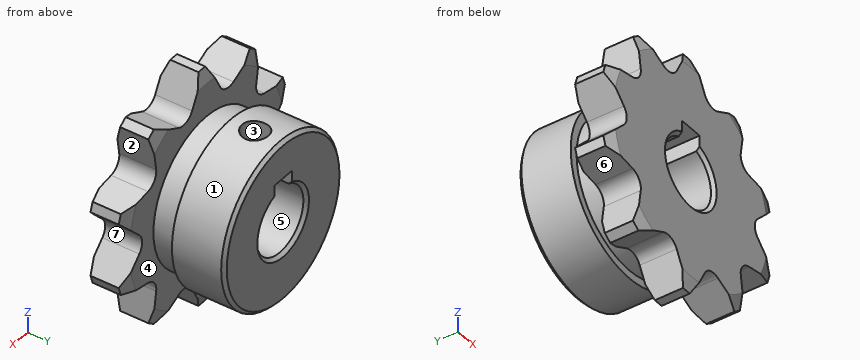
from build123d import *

# Parameters (mm, degrees)
SALIENTE_EXTRUIR1_DEPTH = 7.2136
CROQUIS2_R              = 15.875
SALIENTE_EXTRUIR2_DEPTH = 15.0114
CROQUIS5_R              = 6.35
CORTAR_EXTRUIR2_DEPTH   = 23.2250001
CHAFL_N2_SIZE           = 0.635
REDONDEO1_R             = 0.635
CROQUIS8_W              = 3.175
CROQUIS8_H              = 4.7625
CROQUIS9_W              = 2.5527
CROQUIS9_H              = 15.875
CHAFL_N3_SIZE           = 0.635
CROQUIS11_W             = 4.7625
CROQUIS11_H             = 4.7625
CORTAR_EXTRUIR3_DEPTH   = 23.225


with BuildPart() as part:
    # Croquis1 → Saliente-Extruir1 (new body)
    with BuildSketch(Plane(origin=(0, 0, 0), x_dir=(1, 0, 0), z_dir=(0, 1, 0))):
        with BuildLine():
            Line((12.977610276, 19.417818353), (7.368467037, 16.623783971))
            ThreePointArc((7.368467037, 16.623783971), (5.352847667, 16.474371141), (3.81, 17.78))
            Line((3.81, 17.78), (0.9144, 23.337392972))
            ThreePointArc((0.9144, 23.337392972), (0, 23.3553), (-0.9144, 23.337392972))
            Line((-0.9144, 23.337392972), (-3.81, 17.78))
            ThreePointArc((-3.81, 17.78), (-5.352847667, 16.474371141), (-7.368467037, 16.623783971))
            Line((-7.368467037, 16.623783971), (-12.977610276, 19.417818353))
            ThreePointArc((-12.977610276, 19.417818353), (-13.727900903, 18.894834609), (-14.457140556, 18.342876684))
            Line((-14.457140556, 18.342876684), (-13.533176534, 12.144860349))
            ThreePointArc((-13.533176534, 12.144860349), (-14.013937128, 10.181721309), (-15.732430111, 9.117847487))
            Line((-15.732430111, 9.117847487), (-21.91261452, 8.081297111))
            ThreePointArc((-21.91261452, 8.081297111), (-22.212210255, 7.217184609), (-22.477744799, 6.342004954))
            Line((-22.477744799, 6.342004954), (-18.087139608, 1.870796833))
            ThreePointArc((-18.087139608, 1.870796833), (-17.322178923, 0), (-18.087139608, -1.870796833))
            Line((-18.087139608, -1.870796833), (-22.477744799, -6.342004954))
            ThreePointArc((-22.477744799, -6.342004954), (-22.212210255, -7.217184609), (-21.91261452, -8.081297111))
            Line((-21.91261452, -8.081297111), (-15.732430111, -9.117847487))
            ThreePointArc((-15.732430111, -9.117847487), (-14.013937128, -10.181721309), (-13.533176534, -12.144860349))
            Line((-13.533176534, -12.144860349), (-14.457140556, -18.342876684))
            ThreePointArc((-14.457140556, -18.342876684), (-13.727900903, -18.894834609), (-12.977610276, -19.417818353))
            Line((-12.977610276, -19.417818353), (-7.368467037, -16.623783971))
            ThreePointArc((-7.368467037, -16.623783971), (-5.352847667, -16.474371141), (-3.81, -17.78))
            Line((-3.81, -17.78), (-0.9144, -23.337392972))
            ThreePointArc((-0.9144, -23.337392972), (0, -23.3553), (0.9144, -23.337392972))
            Line((0.9144, -23.337392972), (3.81, -17.78))
            ThreePointArc((3.81, -17.78), (5.352847667, -16.474371141), (7.368467037, -16.623783971))
            Line((7.368467037, -16.623783971), (12.977610276, -19.417818353))
            ThreePointArc((12.977610276, -19.417818353), (13.727900903, -18.894834609), (14.457140556, -18.342876684))
            Line((14.457140556, -18.342876684), (13.533176534, -12.144860349))
            ThreePointArc((13.533176534, -12.144860349), (14.013937128, -10.181721309), (15.732430111, -9.117847487))
            Line((15.732430111, -9.117847487), (21.91261452, -8.081297111))
            ThreePointArc((21.91261452, -8.081297111), (22.212210255, -7.217184609), (22.477744799, -6.342004954))
            Line((22.477744799, -6.342004954), (18.087139608, -1.870796833))
            ThreePointArc((18.087139608, -1.870796833), (17.322178923, 0), (18.087139608, 1.870796833))
            Line((18.087139608, 1.870796833), (22.477744799, 6.342004954))
            ThreePointArc((22.477744799, 6.342004954), (22.212210255, 7.217184609), (21.91261452, 8.081297111))
            Line((21.91261452, 8.081297111), (15.732430111, 9.117847487))
            ThreePointArc((15.732430111, 9.117847487), (14.013937128, 10.181721309), (13.533176534, 12.144860349))
            Line((13.533176534, 12.144860349), (14.457140556, 18.342876684))
            ThreePointArc((14.457140556, 18.342876684), (13.727900903, 18.894834609), (12.977610276, 19.417818353))
        make_face()
    extrude(amount=SALIENTE_EXTRUIR1_DEPTH)

    # Croquis2 → Saliente-Extruir2 (add)
    with BuildSketch(Plane(origin=(0, 7.2136, 0), x_dir=(1, 0, 0), z_dir=(0, 1, 0))):
        Circle(CROQUIS2_R)
    extrude(amount=SALIENTE_EXTRUIR2_DEPTH)

    # Croquis3 → Cortar-Revolución3 (revolve, cut)
    with BuildSketch(Plane(origin=(0, 0, 0), x_dir=(0, 0, -1), z_dir=(1, 0, 0))):
        Polygon((23.972392972, 7.2136), (23.972392972, 6.1468), (20.797392972, 7.2136), align=None)
    cortar_revoluci_n3 = revolve(axis=Axis((0, 0, 0), (0, -1, 0)), mode=Mode.SUBTRACT)

    # Simetría1: Cortar-Revolución3 across plane
    add(cortar_revoluci_n3.mirror(Plane.ZX.offset(3.6068)), mode=Mode.SUBTRACT)

    # Croquis5 → Cortar-Extruir2 (cut, through all)
    with BuildSketch(Plane(origin=(0, 22.225, 0), x_dir=(1, 0, 0), z_dir=(0, 1, 0))):
        Circle(CROQUIS5_R)
    extrude(amount=-CORTAR_EXTRUIR2_DEPTH, mode=Mode.SUBTRACT)

    # Chaflán2
    chafl_n2_edges = [part.edges().sort_by_distance(p)[0] for p in [
        (-15.875, 22.225, 0),
    ]]
    chamfer(chafl_n2_edges, length=CHAFL_N2_SIZE)

    # Redondeo1
    redondeo1_edges = [part.edges().sort_by_distance(p)[0] for p in [
        (-15.875, 7.2136, 0),
    ]]
    fillet(redondeo1_edges, radius=REDONDEO1_R)

    # Croquis8 → Cortar-Revolución4 (revolve, cut)
    with BuildSketch(Plane(origin=(0, 0, 0), x_dir=(0, 0, -1), z_dir=(1, 0, 0))):
        with Locations((-15.870465895, 9.59485)):
            Rectangle(CROQUIS8_W, CROQUIS8_H)
    revolve(axis=Axis((0, 0, -0.004534105), (0, -1, 0)), mode=Mode.SUBTRACT)

    # Croquis9 → Taladro roscado 1/4-201 (revolve, cut)
    with BuildSketch(Plane(origin=(0, 16.78305, 0), x_dir=(0, 1, 0), z_dir=(1, 0, 0))):
        with Locations((1.27635, 7.9375)):
            Rectangle(CROQUIS9_W, CROQUIS9_H)
    revolve(axis=Axis((0, 16.78305, -6.35), (0, 0, 1)), mode=Mode.SUBTRACT)

    # Chaflán3
    chafl_n3_edges = [part.edges().sort_by_distance(p)[0] for p in [
        (-6.35, 0, 0),
        (-6.35, 22.225, 0),
    ]]
    chamfer(chafl_n3_edges, length=CHAFL_N3_SIZE)

    # Croquis11 → Cortar-Extruir3 (cut, through all)
    with BuildSketch(Plane.XZ):
        with Locations((0, 6.35)):
            Rectangle(CROQUIS11_W, CROQUIS11_H)
    extrude(amount=-CORTAR_EXTRUIR3_DEPTH, mode=Mode.SUBTRACT)


solid = part.part
The model under review builds one solid part; all positions refer to its coordinate system, in mm. Face numbers are marked on the shaded views. A direction names the side the tool comes from. Round coordinates to 2 decimals unless told otherwise and drop trailing zeros. Loops run counter-clockwise (first coordinate to the right, second up) from the corner with the lowest first, then second, coordinate; pieces in that order, holes last. Notation, with made-up numbers: (74, 14.25) -> (132, 14.25) arc R17 ccw to (132, 45.25) -> close; hole circle Ø6 at (59, 14.5). An arc over 180 degrees is marked (long way). One line per question, with ' | ' between items. Start each with the question number.
Item 1: For pin 1 (4 mm diameter, centred on y = 11.5, z = 5, fed in from +X); pin 2 (2.5 mm diameter, centred on y = 19, z = 7, fed in from +X); pin 3 (5 mm diameter, centred on x = -0.5, y = 10.5, fed in from -Z) (3 decimals), all flat-tipped, find the tip position at first contact; note any pin that passes through.
Item 2: Machinability: for the marked faces 1, 2 and 3, which of the approach directions +Z, -Z, +X, -X, +Y, -Y give a long, thin tool a straight path to every point of the face, cutting with its end or side? Answer none if there is none.
Item 3: Wall thickness on line 1 along Z through (x, y) = (0, 12.75) (3 decimals); line 2 along X through (y, z) = (11.25, 0); line 3 along Y through (x, z) = (0, 13) (3 decimals): over which ranges is each line inside the solid? List them lowest first. Write a range as [from, to].
Item 4: Draft analysis for pull direction Z (two halves, no side actions). For the marked faces 4, 5, 6 and 7, state which applies: +Z half, -Z half, draft (parallel to the pull), parting line (faces both ways), or undercut.
Item 5: Add section A-A, the plane x = 0. Write out the cut boundary in (y, z) (3 decimals).
Return value:
1) pin 1: stops at x = 15.58 | pin 2: stops at x = 14.8 | pin 3: stops at z = -15.875
2) face 1: +Y | face 2: +X, +Y, -Y | face 3: +Z
3) line 1: z = [-15.875, -6.35], [8.731, 15.875] | line 2: x = [-14.29, -6.35], [6.35, 14.29] | line 3: y = [0, 14.23], [19.336, 22.225]
4) face 4: draft | face 5: undercut | face 6: -Z half | face 7: undercut
5) outline: (0, -20.797) -> (0.859, -23.355) -> (6.354, -23.355) -> (7.214, -20.797) -> (7.214, -14.292) -> (11.976, -14.292) -> (11.976, -15.875) -> (21.59, -15.875) -> (22.225, -15.24) -> (22.225, -6.985) -> (21.59, -6.35) -> (0.635, -6.35) -> (0, -6.985) -> close; (0, 8.731) -> (14.23, 8.731) -> (14.23, 15.875) -> (11.976, 15.875) -> (11.976, 14.283) -> (7.214, 14.283) -> (7.214, 20.797) -> (6.354, 23.355) -> (0.859, 23.355) -> (0, 20.797) -> close; (19.336, 8.731) -> (22.225, 8.731) -> (22.225, 15.24) -> (21.59, 15.875) -> (19.336, 15.875) -> close
